from build123d import *

# Parameters (mm, degrees)
SKETCH1_R           = 3
BOSS_EXTRUDE1_DEPTH = 90
BOSS_EXTRUDE2_DEPTH = 5
FILLET2_R           = 3
SKETCH5_R           = 0.75
CUT_EXTRUDE2_DEPTH  = 92.438503925


with BuildPart() as part:
    # Sketch1 → Boss-Extrude1 (new body)
    with BuildSketch(Plane(origin=(0, 0, 0), x_dir=(1, 0, 0), z_dir=(0, 1, 0))):
        with Locations(Location((0, 0, 0), (0, 0, 270))):
            Circle(SKETCH1_R)
    extrude(amount=-BOSS_EXTRUDE1_DEPTH)

    # Sketch2 → Boss-Extrude2 (add)
    with BuildSketch(Plane(origin=(0, 0, 0), x_dir=(1, 0, 0), z_dir=(0, 1, 0))):
        Polygon((0, 0), (0, 3), (15, 3), (15, -3), (0, -3), align=None)
    extrude(amount=-BOSS_EXTRUDE2_DEPTH)

    # Fillet2
    fillet2_edges = [part.edges().sort_by_distance(p)[0] for p in [
        (15, -5, 0),
    ]]
    fillet(fillet2_edges, radius=FILLET2_R)

    # Sketch5 → Cut-Extrude2 (cut, through all)
    with BuildSketch(Plane.XY.offset(3)):
        with Locations(Location((0, -55, 0), (0, 0, 90))):
            Circle(SKETCH5_R)
    extrude(amount=-CUT_EXTRUDE2_DEPTH, mode=Mode.SUBTRACT)


solid = part.part
For this review, take the finished solid that the model builds, in its own axes (mm). A direction names the side the tool comes from. Give positions to 0.01 mm unless a question says otherwise; leave off trailing zeros. Loops run counter-clockwise (first coordinate to the right, second up) from the corner with the lowest first, then second, coordinate; pieces in that order, holes last. Notation, with made-up numbers: M 15.5,32 L 25.5,32 A8 cw 25.5,40 Z; hole C 16.5,35 d8. An arc over 180 degrees is marked long. Answer as a JSON object with one key per item and string values. Group by question number.
Q1. Insertion check: P1, Ø1, axis at y = -23, z = 1, coming from the +X side; P2, Ø1.5, axis at y = -80, z = 2.5, coming from the +X side; P3, Ø1, axis at y = -67.5, z = -1.5, coming from the -X side; P4, Ø1.2, axis at x = 0, y = -55, coming from the +Z side. Each pin has a flat end and moves straight along its axis. Give the tip position at first contact, or say it passes through.
Q2. For probe 1 along X at (y, z) = (-55, 0); probe 2 along Y at (x, z) = (6.75, 0); probe 3 along Z at (x, y) = (2.75, -14), list the stretches that pass through material, from the lowest coordinate up. Write a range as [from, to].
Q3. Add section C-C on y = -23. Give the boundary of the cut face in (x, z), and give its area (3 significant figures).
Q4. Tool access review of faces 4 (the cylindrical face through (-2.662, -44.37, 1.384)), 5 (the flat face through (6, 0, 0)): name each direction out of +Z, -Z, +X, -X, +Y, -Y from which nothing blocks a thin tool from reaching the whole face with its end or side.
Q5. Add section A-A on z = 0. Give the boundary of the cut face in (x, y), and give its area (3 significant figures).
Q6. Add section B-B on x = 4. Give the boundary of the cut face in (y, z).
Q7. Add section D-D on y = -55. Give the boundary of the cut face in (x, z), and give its area (3 significant figures).
Q8. Mouldability with a two-part tool opening along Y and no side actions: class faces 1 (the flat face through (7, -5, 0)), 2 (the cylindrical face through (-0.03, -55.75, 0.04)), 3 (the flat face through (8, -2, 3)) as +Y half, -Y half, draft (parallel to the pull), parting line (faces both ways), or undercut.
Checked values:
{
 "1": {"P1": "x = 2.96", "P2": "x = 2.44", "P3": "x = -2.83", "P4": "through"},
 "2": {"probe 1": "[-3, -0.75], [0.75, 3]", "probe 2": "[-5, 0]", "probe 3": "[-1.2, 1.2]"},
 "3": {"outline": "C 0,0 d6", "area": "28.3 mm²"},
 "4": {"face 4": "-Y", "face 5": "+Z, -Z, +X, -X, +Y"},
 "5": {"outline": "M -3,-90 L 3,-90 L 3,-5 L 12,-5 A3 ccw 15,-2 L 15,0 L -3,0 Z; hole C 0,-55 d1.5", "area": "596 mm²"},
 "6": {"outline": "M -5,-3 L 0,-3 L 0,3 L -5,3 Z"},
 "7": {"outline": "M -0.75,-2.9 L -0.75,2.9 A3 ccw Z; M 0.75,-2.9 A3 ccw 0.75,2.9 Z", "area": "19.4 mm²"},
 "8": {"face 1": "-Y half", "face 2": "undercut", "face 3": "draft"}
}
